from build123d import *

# Parameters (mm, degrees)
CUT_EXTRUDE_1_DEPTH      = 67.426651278
CUT_EXTRUDE_1_DEPTH_BACK = 67.426651278
SKETCH_2_R               = 4
SKETCH_3_R               = 5.5
CUT_EXTRUDE_2_DEPTH      = 7


with BuildPart() as part:
    # ｽｹｯﾁ1 → 回転1 (revolve)
    with BuildSketch(Plane.XY, mode=Mode.PRIVATE) as revolve_1_sk:
        Polygon((-40, 16.5), (-5, 16.5), (-5, 13), (0, 13), (0, 37.5), (-40, 37.5), align=None)
    revolve(revolve_1_sk.sketch.rotate(Axis((-40, 0, 0), (1, 0, 0)), 90), axis=Axis((-40, 0, 0), (1, 0, 0)))

    # ｽｹｯﾁ2 → ｶｯﾄ - 押し出し1 (cut, two sides: drawn at the far end of the back side and taken through both)
    with BuildSketch(Plane(origin=(0, 0, 0), x_dir=(0, 0, -1), z_dir=(1, 0, 0)).offset(-CUT_EXTRUDE_1_DEPTH_BACK)):
        with Locations((30, 0)):
            Circle(SKETCH_2_R)
        with Locations((-30, 0)):
            Circle(SKETCH_2_R)
    extrude(amount=CUT_EXTRUDE_1_DEPTH + CUT_EXTRUDE_1_DEPTH_BACK, mode=Mode.SUBTRACT)

    # ｽｹｯﾁ3 → ｶｯﾄ - 押し出し2 (cut)
    with BuildSketch(Plane(origin=(0, 0, 0), x_dir=(0, 0, -1), z_dir=(1, 0, 0))):
        with Locations((30, 0)):
            Circle(SKETCH_3_R)
        with Locations((-30, 0)):
            Circle(SKETCH_3_R)
    extrude(amount=-CUT_EXTRUDE_2_DEPTH, mode=Mode.SUBTRACT)


solid = part.part
Input: part model. Units: mm. Frame: model coordinates. A direction names the side the tool comes from. Give positions to 0.01 mm unless a question says otherwise; leave off trailing zeros. Write each loop counter-clockwise with the first axis right and the second up, starting at its lowest first coordinate (ties: lowest second). Pieces come first, ordered by that corner, then holes. Notation, with made-up numbers: (72, 49) -> (122, 49) arc R27 ccw to (122, 65) -> close; hole circle Ø11 at (68.5, -9). An arc over 180 degrees is marked (long way). Use one line per item in the form item = value. Start each with the question number.
1) Section query B-B on y = 0. Return the cut outline in (x, z), then the cut area to 3 significant figures.
2) Section query A-A on z = -27.5. Return the cut outline in (x, y), then the cut area to 3 significant figures.
3) Set-up query: faces 1 (the cylindrical face through (-23.7, -2.4, -26.8)), 2 (the flat face through (-5, 13.4, -0.1)), 3 (the cylindrical face through (-3.451, 0.242, -24.505)). Return all of +Z, -Z, +X, -X, +Y, -Y with unobstructed straight access to the full face (end or side cutting, diameter ignored); none if empty.
4) Ray query, probe 1 along Y at (x, z) = (-1.85, 0); probe 2 along Z at (x, y) = (-10.5, -1.5); probe 3 along Z at (x, y) = (-4, -5). Return the intervals inside material, ascending. Write a range as from..to.
5) Pin query (flat end, axial travel): pin 1 (3 mm diameter, centred on x = -29, z = 5.5, fed in from +Y); pin 2 (10 mm diameter, centred on y = -7.5, z = 4.5, fed in from -X); pin 3 (5 mm diameter, centred on x = -7.5, z = 15, fed in from +Y). Return the tip coordinate at first contact, or that it passes through.
6) Section query C-C on x = -8. Return the cut outline in (y, z).
7) Section query D-D on z = 0. Return the cut outline in (x, y), then the cut area to 4 significant figures.
Outcome:
q1.outline = (-40, -37.5) -> (0, -37.5) -> (0, -35.5) -> (-7, -35.5) -> (-7, -34) -> (-40, -34) -> close; (-40, -26) -> (-7, -26) -> (-7, -24.5) -> (0, -24.5) -> (0, -13) -> (-5, -13) -> (-5, -16.5) -> (-40, -16.5) -> close; (-40, 16.5) -> (-5, 16.5) -> (-5, 13) -> (0, 13) -> (0, 24.5) -> (-7, 24.5) -> (-7, 26) -> (-40, 26) -> close; (-40, 34) -> (-7, 34) -> (-7, 35.5) -> (0, 35.5) -> (0, 37.5) -> (-40, 37.5) -> close
q1.area = 1,030 mm^2
q2.outline = (-40, -25.5) -> (0, -25.5) -> (0, -4.9) -> (-7, -4.9) -> (-7, -3.12) -> (-40, -3.12) -> close; (-40, 3.12) -> (-7, 3.12) -> (-7, 4.9) -> (0, 4.9) -> (0, 25.5) -> (-40, 25.5) -> close
q2.area = 1,760 mm^2
q3.face_1 = +X, -X
q3.face_2 = -X
q3.face_3 = +X
q4.probe_1 = -37.5..-13, 13..37.5
q4.probe_2 = -37.47..-33.71, -26.29..-16.43, 16.43..26.29, 33.71..37.47
q4.probe_3 = -37.17..-32.29, -27.71..-12, 12..27.71, 32.29..37.17
q5.pin_1 = 37.29
q5.pin_2 = -5
q5.pin_3 = 35.36
q6.outline = circle Ø75 at (0, 0); hole circle Ø33 at (0, 0); hole circle Ø8 at (0, -30); hole circle Ø8 at (0, 30)
q7.outline = (-40, -37.5) -> (0, -37.5) -> (0, -13) -> (-5, -13) -> (-5, -16.5) -> (-40, -16.5) -> close; (-40, 16.5) -> (-5, 16.5) -> (-5, 13) -> (0, 13) -> (0, 37.5) -> (-40, 37.5) -> close
q7.area = 1,715 mm^2
